from build123d import *

# Parameters (mm, degrees)
SKETCH1_R               = 8.9
BOSS_EXTRUDE1_DEPTH     = 2
SKETCH2_R               = 5.9
BOSS_EXTRUDE2_DEPTH     = 20
CUT_EXTRUDE1_DEPTH      = 26.346005602
CUT_EXTRUDE1_DEPTH_BACK = 26.346005602
SKETCH4_W               = 2
SKETCH4_H               = 1
CUT_EXTRUDE2_DEPTH      = 1.2
FILLET1_R               = 0.25
FILLET2_R               = 0.25


with BuildPart() as part:
    # Sketch1 → Boss-Extrude1 (new body)
    with BuildSketch(Plane(origin=(0, 0, 0), x_dir=(1, 0, 0), z_dir=(0, 1, 0))):
        with Locations(Location((0, 0, 0), (0, 0, 270))):
            Circle(SKETCH1_R)
    extrude(amount=BOSS_EXTRUDE1_DEPTH)

    # Sketch2 → Boss-Extrude2 (add)
    with BuildSketch(Plane(origin=(0, 2, 0), x_dir=(1, 0, 0), z_dir=(0, 1, 0))):
        with Locations(Location((0, 0, 0), (0, 0, 270))):
            Circle(SKETCH2_R)
    extrude(amount=BOSS_EXTRUDE2_DEPTH)

    # Sketch3 → Cut-Extrude1 (cut, two sides: drawn at the far end of the back side and taken through both)
    with BuildSketch(Plane.XY.offset(-CUT_EXTRUDE1_DEPTH_BACK)):
        Polygon((-6.28, 5.42), (6.28, 17.98), (6.28, 28.771900514), (-6.28, 28.771900514), align=None)
    extrude(amount=CUT_EXTRUDE1_DEPTH + CUT_EXTRUDE1_DEPTH_BACK, mode=Mode.SUBTRACT)

    # Sketch4 → Cut-Extrude2 (cut)
    with BuildSketch(Plane.XZ):
        with Locations((4, 0)):
            Rectangle(SKETCH4_W, SKETCH4_H)
    extrude(amount=-CUT_EXTRUDE2_DEPTH, mode=Mode.SUBTRACT)

    # Fillet1
    fillet1_edges = [part.edges().sort_by_distance(p)[0] for p in [
        (3, 1.2, 0),
        (3, 0.6, -0.5),
        (4, 1.2, 0.5),
        (3, 0.6, 0.5),
        (5, 1.2, 0),
        (5, 0.6, 0.5),
        (4, 1.2, -0.5),
        (5, 0.6, -0.5),
        (3, 0, 0),
        (4, 0, -0.5),
        (5, 0, 0),
        (4, 0, 0.5),
    ]]
    fillet(fillet1_edges, radius=FILLET1_R)

    # Fillet2
    fillet2_edges = [part.edges().sort_by_distance(p)[0] for p in [
        (0, 2, -5.9),
    ]]
    fillet(fillet2_edges, radius=FILLET2_R)


solid = part.part
Part model, mm, in its own coordinate system. A direction names the side the tool comes from. Give positions to 0.01 mm unless a question says otherwise; leave off trailing zeros. Order: outer loops, then holes, each group sorted by start corner. A loop starts at its lowest first (then second) coordinate and runs counter-clockwise, first axis right, second up. Notation, with made-up numbers: (-6, -25.5) - (28, -25.5) arc R4 cw to (28, -21.5) - close; hole circle Ø11 at (15, 81). An arc over 180 degrees is marked (long way). One line per question, with ' | ' between items.
1. Band-saw the part on B-B on x = 0. List the corners of the cut face in (y, z).
Filled in:
outline: (0, -8.9) - (2, -8.9) - (2, -6.15) arc R0.25 cw to (2.25, -5.9) - (11.7, -5.9) - (11.7, 5.9) - (2.25, 5.9) arc R0.25 cw to (2, 6.15) - (2, 8.9) - (0, 8.9) - close
2. Band-saw the part on C-C on y = 8. List the corners of the cut face in (x, z).
Filled in:
outline: (-3.7, -4.6) arc R5.9 ccw (long way) to (-3.7, 4.6) - close
3. Drill centre lines: probe 1 along X at (y, z) = (4, -0.5); probe 2 along X at (y, z) = (5, -5); probe 3 along Y at (x, z) = (-2.25, 5.5). Where is each one in solid material? Low to high.
Filled in:
probe 1: -5.88 to 5.88 | probe 2: -3.13 to 3.13 | probe 3: 0 to 2.11
4. Band-saw the part on A-A on z = 0. List the corners of the cut face in (x, y), then the cut area to 3 significant figures.
Filled in:
outline: (-8.9, 0) - (2.75, 0) arc R0.25 ccw to (3, 0.25) - (3, 0.95) arc R0.25 cw to (3.25, 1.2) - (4.75, 1.2) arc R0.25 cw to (5, 0.95) - (5, 0.25) arc R0.25 ccw to (5.25, 0) - (8.9, 0) - (8.9, 2) - (6.15, 2) arc R0.25 cw to (5.9, 2.25) - (5.9, 17.6) - (-5.9, 5.8) - (-5.9, 2.25) arc R0.25 cw to (-6.15, 2) - (-8.9, 2) - close | area: 148 mm²
5. Which spindle directions (+Z, -Z, +X, -X, +Y, -Y) get a long thin tool onto all of the face, cutting with end or side? Do faces 1 (the face through (-6, 2, -2)), 2 (the face through (0, 0, 0)). Say none if no direction does.
Filled in:
face 1: +Y | face 2: +Z, -Z, +X, -X, -Y
6. Band-saw the part on D-D on y = 4.5. List the corners of the cut face in (x, z).
Filled in:
outline: circle Ø11.8 at (0, 0)
7. Drop flat-ended pins along their axis: P1, Ø2, axis at y = 14.5, z = 3.5, coming from the +X side; P2, Ø10, axis at x = -5, y = 13.5, coming from the -Z side; P3, Ø3, axis at y = 15.5, z = 4.5, coming from the -X side. Give the stop position or say it passes through.
Filled in:
P1: x = 5.34 | P2: z = -5.87 | P3: x = 2.3
